The model under review builds one solid part; all positions refer to its coordinate system, in mm. A direction names the side the tool comes from. Give positions to 0.01 mm unless a question says otherwise; leave off trailing zeros. Order: outer loops, then holes, each group sorted by start corner. A loop starts at its lowest first (then second) coordinate and runs counter-clockwise, first axis right, second up. Notation, with made-up numbers: (66, 36.5) - (93, 36.5) arc R26 cw to (93, 70.5) - close; hole circle Ø7 at (-17, 89.5). An arc over 180 degrees is marked (long way). Write item = value, one per line. Start each with the question number.
1. We need section D-D, the plane y = 22. Give the boundary of the cut face in (x, z).
2. For P1, Ø1, axis at y = -2, z = -545, coming from the +X side; P2, Ø1, axis at x = 353, z = -258, coming from the -Y side; P3, Ø5, axis at x = 803, y = -56.5, coming from the +Z side, all flat-tipped, find the tip position at first contact; note any pin that passes through.
3. We need section B-B, the plane z = -760.5. Give the boundary of the cut face in (x, y), and give its area (3 significant figures).
4. We need section A-A, the plane x = 667.5. Give the boundary of the cut face in (y, z), and give its area (3 significant figures).
5. Mouldability with a two-part tool opening along Z and no side actions: class faces 1 (the flat face through (592, 50, -493)), 2 (the flat face through (592, 25, 0)), 3 (the flat face through (872, 25, -75)), 4 (the flat face through (322, 25, -900)) as pulls with the +Z half, pulls with the -Z half, needs draft (parallel to the pull), parting line crosses it, or undercut.
6. We need section C-C, the plane x = 266.5. Give the boundary of the cut face in (y, z), and give its area (3 significant figures).
7. Machinability: for faces 5 (the flat face through (322, 25, -275)), 6 (the flat face through (608, -11, -1000)), which of the approach directions +Z, -Z, +X, -X, +Y, -Y give a long, thin tool a straight path to every point of the face, cutting with its end or side? Answer none if there is none.
8. Wall thickness on probe 1 along X at (y, z) = (32.5, -509); probe 2 along Z at (x, y) = (817, 39.5); probe 3 along Y at (x, z) = (705, -45): over which ranges is each line inside the solid? List them lowest first.
from build123d import *

# Parameters (mm, degrees)
F0_W     = 1200
F0_H     = 1000
F0_W_2   = 500
F0_H_2   = 625
F0_H_3   = 150
F0_H_4   = 825
F1_DEPTH = 50
F3_DEPTH = 1200


with BuildPart() as f1:
    # F0 (on Front) → F1 (new body)
    with BuildSketch(Plane.XZ):
        with Locations((600, -500)):
            Rectangle(F0_W, F0_H)
        with Locations((325, -587.5)):
            Rectangle(F0_W_2, F0_H_2, mode=Mode.SUBTRACT)
        with Locations((325, -150)):
            Rectangle(F0_W_2, F0_H_3, mode=Mode.SUBTRACT)
        with Locations((875, -487.5)):
            Rectangle(F0_W_2, F0_H_4, mode=Mode.SUBTRACT)
    extrude(amount=-F1_DEPTH)

    # F2 (on face) → F3 (join)
    with BuildSketch(Plane.YZ.offset(1200)):
        Polygon((-70, -1000), (0, -1000), (0, -962.657111), (-70, -975), align=None)
    extrude(amount=-F3_DEPTH)


solid = f1.part
Model answer:
q1.outline = (0, -1000) - (1200, -1000) - (1200, 0) - (0, 0) - close; hole (75, -900) - (575, -900) - (575, -275) - (75, -275) - close; hole (75, -225) - (575, -225) - (575, -75) - (75, -75) - close; hole (625, -900) - (1125, -900) - (1125, -75) - (625, -75) - close
q2.P1 = through
q2.P2 = 0
q2.P3 = -972.18
q3.outline = (0, 0) - (75, 0) - (75, 50) - (0, 50) - close; (575, 0) - (625, 0) - (625, 50) - (575, 50) - close; (1125, 0) - (1200, 0) - (1200, 50) - (1125, 50) - close
q3.area = 10,000 mm2
q4.outline = (-70, -1000) - (50, -1000) - (50, -900) - (0, -900) - (0, -962.66) - (-70, -975) - close; (0, -75) - (50, -75) - (50, 0) - (0, 0) - close
q4.area = 10,900 mm2
q5.face_1 = needs draft
q5.face_2 = pulls with the +Z half
q5.face_3 = undercut
q5.face_4 = undercut
q6.outline = (-70, -1000) - (50, -1000) - (50, -900) - (0, -900) - (0, -962.66) - (-70, -975) - close; (0, -275) - (50, -275) - (50, -225) - (0, -225) - close; (0, -75) - (50, -75) - (50, 0) - (0, 0) - close
q6.area = 13,400 mm2
q7.face_5 = +Y, -Y
q7.face_6 = -Z, +X, -X, +Y, -Y
q8.probe_1 = 0 to 75, 575 to 625, 1125 to 1200
q8.probe_2 = -1000 to -900, -75 to 0
q8.probe_3 = 0 to 50
